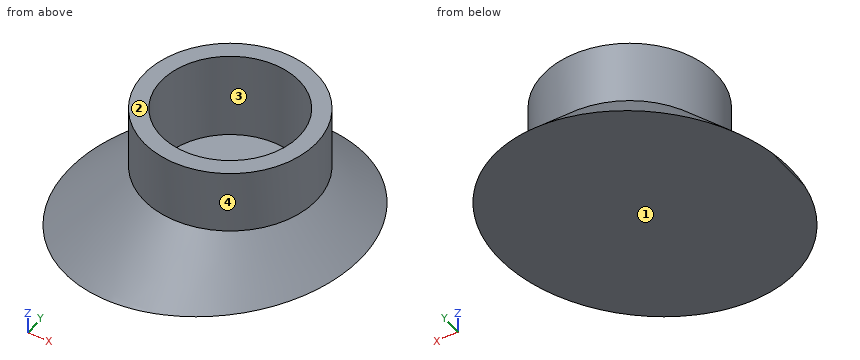
from build123d import *

# Parameters (mm, degrees)
F2_R     = 12
F3_DEPTH = 15
F5_DEPTH = 50


with BuildPart() as f1:
    # F0 (on Front) → F1 (revolve)
    with BuildSketch(Plane.XZ):
        Polygon((0, 24), (0, 0), (28, 0), (15, 13), (15, 24), align=None)
    revolve(axis=Axis((0, 0, 12), (0, 0, -1)))

    # F2 (on face) → F3 (cut)
    with BuildSketch(Plane.XY.offset(24)):
        Circle(F2_R)
    extrude(amount=-F3_DEPTH, mode=Mode.SUBTRACT)

    # F4 (on Front) → F5 (cut, symmetric)
    with BuildSketch(Plane.XZ):
        Polygon((33.364898, 6.410917), (-27.630899, 0), (33.364898, 0), align=None)
    extrude(amount=F5_DEPTH, both=True, mode=Mode.SUBTRACT)


solid = f1.part
Geometry check sheet. Reference: the model listing, model coordinates, mm. Face numbers are marked on the shaded views. Round coordinates to 2 decimals unless told otherwise and drop trailing zeros. Write each loop counter-clockwise with the first axis right and the second up, starting at its lowest first coordinate (ties: lowest second). Pieces come first, ordered by that corner, then holes.
Item 1: Mould release check, pull along X, two halves, no side actions. Record for the marked faces 1, 2, 3 and 4: +X half, -X half, draft (parallel to the pull), parting line (faces both ways), or undercut.
Determined:
face 1: +X half
face 2: draft
face 3: undercut
face 4: parting line
Item 2: Section check D-D (z = 6.5). Record the boundary of the cut face in (x, y), plus the area to 3 significant figures.
Determined:
outline: circle Ø43 at (0, 0)
area: 1,450 mm2
Item 3: Section check A-A (y = 0). Record the boundary of the cut face in (x, z), plus the area to 3 significant figures.
Determined:
outline: (-28, 0) - (-27.63, 0) - (22.71, 5.29) - (15, 13) - (15, 24) - (12, 24) - (12, 9) - (-12, 9) - (-12, 24) - (-15, 24) - (-15, 13) - close
area: 382 mm2
Item 4: Section check B-B (z = 14.25). Record the boundary of the cut face in (x, y).
Determined:
outline: circle Ø30 at (0, 0); hole circle Ø24 at (0, 0)
Item 5: Section check C-C (x = 0). Record the boundary of the cut face in (y, z).
Determined:
outline: (-25.1, 2.9) - (25.1, 2.9) - (15, 13) - (15, 24) - (12, 24) - (12, 9) - (-12, 9) - (-12, 24) - (-15, 24) - (-15, 13) - close
Item 6: Material ranges on line 1 along Y through (x, z) = (0, 18.25); line 2 along X through (y, z) = (6.5, 13); line 3 along Y through (x, z) = (2, 10), recorded low to high.
Determined:
line 1: y = -15 to -12, 12 to 15
line 2: x = -13.52 to -10.09, 10.09 to 13.52
line 3: y = -17.89 to -11.83, 11.83 to 17.89
Item 7: Go/stop test with flat-tipped pins: pin 1 Ø8 at (x, y) = (7.5, -18) entering from -Z; pin 2 Ø3 at (y, z) = (-9, 10.5) entering from +X; pin 3 Ø8 at (x, y) = (10, -18.5) entering from +Z. Record where each tip stops, or that it passes through.
Determined:
pin 1: stops at z = 3.27
pin 2: stops at x = 16.9
pin 3: stops at z = 10.97
